```python
from build123d import *

# Parameters (mm, degrees)
BOSS_EXTRUDE1_DEPTH = 33
SKETCH2_R           = 10.65
CUT_EXTRUDE1_DEPTH  = 10


with BuildPart() as part:
    # Sketch1 → Boss-Extrude1 (new body)
    with BuildSketch(Plane(origin=(0, 0, 0), x_dir=(-1, 0, 0), z_dir=(0, 1, 0))):
        with BuildLine():
            Line((15.705832049, -67.814850439), (39.165320565, -67.814850439))
            ThreePointArc((39.165320565, -67.814850439), (27.435576307, -15.429277781), (15.705832049, -67.814850439))
        make_face()
        with BuildLine():
            Line((15.935576307, -66.798850439), (38.935576307, -66.798850439))
            ThreePointArc((38.935576307, -66.798850439), (27.435576307, -16.445277781), (15.935576307, -66.798850439))
        make_face(mode=Mode.SUBTRACT)
    extrude(amount=BOSS_EXTRUDE1_DEPTH)

    # Sketch2 → Cut-Extrude1 (cut)
    with BuildSketch(Plane(origin=(0, 0, -67.814850439), x_dir=(-1, 0, 0), z_dir=(0, 0, -1))):
        with Locations((27.435576307, 18.5)):
            Circle(SKETCH2_R)
    extrude(amount=-CUT_EXTRUDE1_DEPTH, mode=Mode.SUBTRACT)


solid = part.part
```
Design review of the part built by this model. Coordinates are the model's own, in mm. A direction names the side the tool comes from. Round coordinates to 2 decimals unless told otherwise and drop trailing zeros. Order: outer loops, then holes, each group sorted by start corner. A loop starts at its lowest first (then second) coordinate and runs counter-clockwise, first axis right, second up. Notation, with made-up numbers: M 8,-20.75 L 23,-20.75 A23 cw 23,-3.75 Z; hole C 80.25,-1.75 d8. An arc over 180 degrees is marked long. Put each result on its own line as item: value.
Q1. Consider section A-A (x = -33). State the section outline as (y, z) points, and give its area (3 significant figures).
Reported:
outline: M 0,-67.81 L 9.42,-67.81 L 9.42,-66.8 L 0,-66.8 Z; M 0,-17.04 L 33,-17.04 L 33,-16 L 0,-16 Z; M 27.58,-67.81 L 33,-67.81 L 33,-66.8 L 27.58,-66.8 Z
area: 49.3 mm²
Q2. Insertion check: pin 1 Ø12 at (x, y) = (-21, 20.5) entering from +Z; pin 2 Ø12 at (x, y) = (-48.5, 4) entering from +Z; pin 3 Ø3 at (x, z) = (-46.5, -29) entering from -Y; pin 4 Ø5 at (y, z) = (13.5, -25) entering from -X. Each pin has a flat end and moves straight along its axis. Give the tip position at first contact, or say it passes through.
Reported:
pin 1: z = -15.43
pin 2: z = -19.92
pin 3: through
pin 4: x = -50.2
Q3. To check wall thickness, follow line 1 (Z direction, x = -7, y = 23); line 2 (X direction, y = 25, z = -46.5); line 3 (X direction, y = 19, z = -64.5). State the ranges of each line that lie inside material, in increasing order.
Reported:
line 1: -61.35 to -59.79, -26.08 to -24.52
line 2: -54.71 to -53.68, -1.19 to -0.16
line 3: -44.51 to -42.82, -12.05 to -10.36
Q4. Consider section D-D (x = -46.5). State the section outline as (y, z) points.
Reported:
outline: M 0,-62.76 L 33,-62.76 L 33,-61.33 L 0,-61.33 Z; M 0,-24.54 L 33,-24.54 L 33,-23.11 L 0,-23.11 Z
Q5. Draft analysis for pull direction Z (two halves, no side actions). For faces 3 (the face through (-32.4, 8.9, -66.799)), 4 (the face through (-22, 9, -67.815)), 5 (the face through (-13, 33, -20)), state which applies: released by +Z, released by -Z, zero draft, split by the parting line, or undercut.
Reported:
face 3: undercut
face 4: released by -Z
face 5: zero draft
Q6. Consider section C-C (y = 18.5). State the section outline as (x, z) points, and give its area (3 significant figures).
Reported:
outline: M -39.17,-67.81 L -38.09,-67.81 L -38.09,-66.8 L -38.94,-66.8 A26.49 cw long -15.94,-66.8 L -16.79,-66.8 L -16.79,-67.81 L -15.71,-67.81 A27.51 ccw long Z
area: 150 mm²
Q7. Machinability: for faces 1 (the face through (-28.434, 16.269, -16.464)), 2 (the face through (-37.594, 21.699, -67.314)), which of the approach directions +Z, -Z, +X, -X, +Y, -Y give a long, thin tool a straight path to every point of the face, cutting with its end or side? Answer none if there is none.
Reported:
face 1: +Y, -Y
face 2: -Z
Q8. Consider section B-B (z = -24). State the section outline as (x, y) points.
Reported:
outline: M -47.39,0 L -45.96,0 L -45.96,33 L -47.39,33 Z; M -8.91,0 L -7.48,0 L -7.48,33 L -8.91,33 Z
